Check sheet for the drawn part. Datum: minimum x, y, z corner. Units: mm. A direction names the side the tool comes from. Coordinates: 2 decimals unless noted, no trailing zeros. Write each loop counter-clockwise with the first axis right and the second up, starting at its lowest first coordinate (ties: lowest second). Pieces come first, ordered by that corner, then holes. Notation, with made-up numbers: M -35.75,23 L -20.75,23 A27 ccw -20.75,56 Z; hole C -2.75,70 d11. An arc over 180 degrees is marked long. Answer as a JSON object with one key per item and string values. Group by question number.
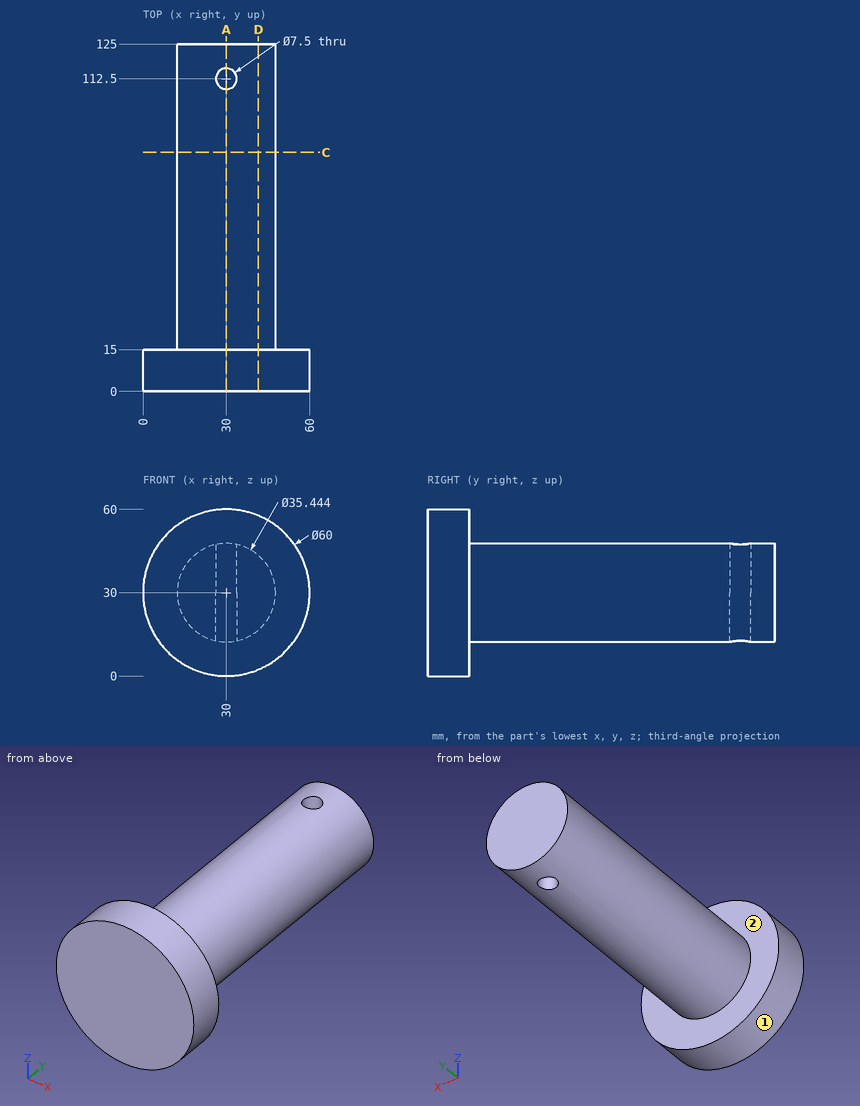
1) Go/stop test with flat-tipped pins: pin 1 Ø10 at (x, y) = (30, 112.5) entering from +Z; pin 2 Ø6 at (x, z) = (50.5, 15) entering from +Y; pin 3 Ø10 at (x, y) = (13.5, 75) entering from +Z (1 decimal). Record where each tip stops, or that it passes through.
2) Section check A-A (x = 30). Record the cut outline in (y, z), then the cut area to 3 significant figures.
3) Set-up check for the marked faces 1 and 2: record each of +Z, -Z, +X, -X, +Y, -Y from which the full face is reachable in a straight line by a thin tool's end or side.
4) Material ranges on probe 1 along Y at (x, z) = (30, 18); probe 2 along Y at (x, z) = (3, 26); probe 3 along Z at (x, y) = (31, 107.5), recorded low to high. Write a range as [from, to].
5) Section check C-C (y = 86). Record the cut outline in (x, z) (1 decimal), then the cut area to 3 significant figures.
6) Section check D-D (x = 41.5). Record the cut outline in (y, z) (1 decimal), then the cut area to 3 significant figures.
Entries:
{
 "1": {"pin 1": "z = 47.72", "pin 2": "y = 15", "pin 3": "z = 43.5"},
 "2": {"outline": "M 0,0 L 15,0 L 15,12.28 L 108.75,12.28 L 108.75,47.72 L 15,47.72 L 15,60 L 0,60 Z; M 116.25,12.28 L 125,12.28 L 125,47.72 L 116.25,47.72 Z", "area": "4,530 mm^2"},
 "3": {"face 1": "+Y, -Y", "face 2": "+Y"},
 "4": {"probe 1": "[0, 108.75], [116.25, 125]", "probe 2": "[0, 15]", "probe 3": "[12.31, 47.69]"},
 "5": {"outline": "C 30,30 d35.4", "area": "987 mm^2"},
 "6": {"outline": "M 0,2.3 L 15,2.3 L 15,16.5 L 125,16.5 L 125,43.5 L 15,43.5 L 15,57.7 L 0,57.7 Z", "area": "3,800 mm^2"}
}
